from build123d import *

# Parameters (mm, degrees)
F1_DEPTH = 76.2
F4_DEPTH = 114.301
F5_DEPTH = 114.301
F6_W     = 48.55076
F6_H     = 23.712237
F6_H_2   = 24.714869
F7_DEPTH = 19.051
F8_R     = 8.936908
F9_DEPTH = 19.051


with BuildPart() as f1:
    # F0 (on Front) → F1 (new body)
    with BuildSketch(Plane.XZ):
        Polygon((-30.005424, 30.119236), (-49.055424, 30.119236), (-49.055424, -33.380764), (65.244576, -33.380764), (65.244576, -14.330764), (-30.005424, -14.330764), align=None)
    extrude(amount=F1_DEPTH)

    # F3 (on face) → F4 (cut, through all)
    with BuildSketch(Plane(origin=(-49.055424, 0, 0), x_dir=(0, -1, 0), z_dir=(-1, 0, 0))):
        Polygon((76.2, 0), (76.2, 30.119236), (50.347358, 30.119236), align=None)
    extrude(amount=-F4_DEPTH, mode=Mode.SUBTRACT)

    # F2 (on face) → F5 (cut, through all)
    with BuildSketch(Plane(origin=(-49.055424, 0, 0), x_dir=(0, -1, 0), z_dir=(-1, 0, 0))):
        Polygon((76.2, 30.119236), (50.347358, 30.119236), (76.2, 0), align=None)
    extrude(amount=-F5_DEPTH, mode=Mode.SUBTRACT)

    # F6 (on face) → F7 (cut, through all)
    with BuildSketch(Plane.XY.offset(-14.330764)):
        with Locations((40.969196, -49.956119)):
            Rectangle(F6_W, F6_H)
        with Locations((40.969196, -25.742566)):
            Rectangle(F6_W, F6_H_2)
    extrude(amount=-F7_DEPTH, mode=Mode.SUBTRACT)

    # F8 (on face) → F9 (cut, through all)
    with BuildSketch(Plane.XY.offset(-14.330764)):
        with Locations((-7.438298, -37.598684)):
            Circle(F8_R)
    extrude(amount=-F9_DEPTH, mode=Mode.SUBTRACT)


solid = f1.part
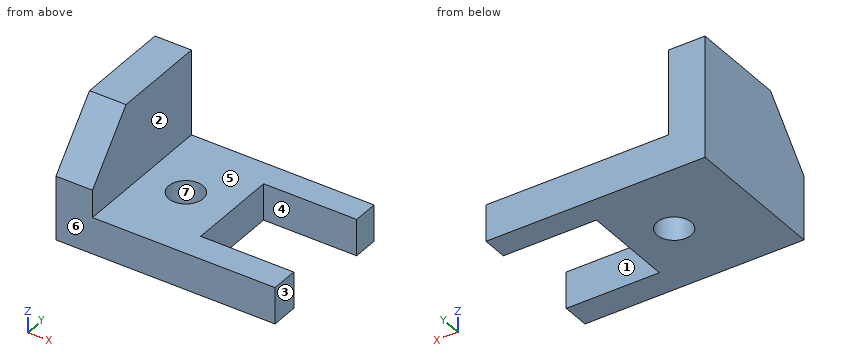
The listing builds one solid part. Answer for the finished solid, in the listing's coordinates (mm). Face numbers are marked on the shaded views. A direction names the side the tool comes from. Coordinates: 2 decimals unless noted, no trailing zeros. Order: outer loops, then holes, each group sorted by start corner. A loop starts at its lowest first (then second) coordinate and runs counter-clockwise, first axis right, second up. Notation, with made-up numbers: M 80.5,-33 L 121.5,-33 A16 cw 121.5,-3 Z; hole C -34,-25 d11. An arc over 180 degrees is marked long. Use CSV: the item, a comma, the result in double quotes.
Q1. Section C-C (y = -21.5) is taken. Determine the outline of the cut face in (x, z), then the cut area to 3 significant figures.
Here are the results:
outline,"M -49.06,-33.38 L 16.69,-33.38 L 16.69,-14.33 L -30.01,-14.33 L -30.01,30.12 L -49.06,30.12 Z"
area,"2,100 mm2"
Q2. Given pin 1 Ø15 at (y, z) = (-43.5, -20.5) entering from +X; pin 2 Ø23 at (x, y) = (8, -19.5) entering from +Z, each flat-ended and moving along its own axis, determine where each tip first touches the part or whether it passes through.
Here are the results:
pin 1,"x = 16.69"
pin 2,"z = -14.33"
Q3. Section B-B (y = -33) is taken. Determine the outline of the cut face in (x, z).
Here are the results:
outline,"M -49.06,-33.38 L -15.1,-33.38 L -15.1,-14.33 L -30.01,-14.33 L -30.01,30.12 L -49.06,30.12 Z; M 0.22,-33.38 L 16.69,-33.38 L 16.69,-14.33 L 0.22,-14.33 Z"
Q4. Straight lines are drawn through the part: L1, parallel to Y at x = 37, z = -30; L2, parallel to Z at x = 0, y = -31.5; L3, parallel to X at y = -5, z = 24. For each, find the intervals that lie inside material, in ascending order.
Here are the results:
L1,"-76.2 to -61.81, -13.39 to 0"
L2,"-33.38 to -14.33"
L3,"-49.06 to -30.01"
Q5. Section D-D (z = -20) is taken. Determine the outline of the cut face in (x, y), then the cut area to 3 significant figures.
Here are the results:
outline,"M -49.06,-76.2 L 65.24,-76.2 L 65.24,-61.81 L 16.69,-61.81 L 16.69,-13.39 L 65.24,-13.39 L 65.24,0 L -49.06,0 Z; hole C -7.44,-37.6 d17.87"
area,"6,110 mm2"
Q6. A tool of negligible diameter and unlimited length cuts with its end or side. For the marked faces 1, 2 and 3, from which of +Z, -Z, +X, -X, +Y, -Y can it reach the whole face along a straight path? Write none if from no direction.
Here are the results:
face 1,"+Z, -Z, +X"
face 2,"+Z, +X, +Y, -Y"
face 3,"+Z, -Z, +X, +Y, -Y"
Q7. Section A-A (x = 48) is taken. Determine the outline of the cut face in (y, z).
Here are the results:
outline,"M -76.2,-33.38 L -61.81,-33.38 L -61.81,-14.33 L -76.2,-14.33 Z; M -13.39,-33.38 L 0,-33.38 L 0,-14.33 L -13.39,-14.33 Z"
Q8. Determine the mould class of the marked faces 4, 5, 6 and 7 for opening direction Y: pulls with the +Y half, pulls with the -Y half, needs draft (parallel to the pull), parting line crosses it, or undercut.
Here are the results:
face 4,"undercut"
face 5,"needs draft"
face 6,"pulls with the -Y half"
face 7,"undercut"
